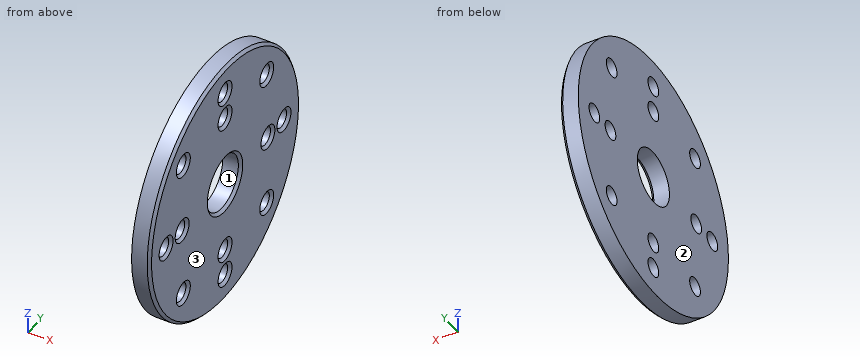
```python
from build123d import *

# Parameters (mm, degrees)
SKETCH1_W          = 2
SKETCH1_H          = 11
SKETCH2_R          = 1
CUT_EXTRUDE1_DEPTH = 20.899748742
CIRPATTERN2_COUNT  = 8
SKETCH3_R          = 1
CUT_EXTRUDE2_DEPTH = 20.899748742
CIRPATTERN3_COUNT  = 4
CHAMFER1_SIZE      = 0.3


with BuildPart() as part:
    # Sketch1 → Revolve1 (revolve)
    with BuildSketch(Plane.XY, mode=Mode.PRIVATE) as revolve1_sk:
        with Locations((-1, 8.5)):
            Rectangle(SKETCH1_W, SKETCH1_H)
    revolve(revolve1_sk.sketch.rotate(Axis((0, 0, 0), (1, 0, 0)), 90), axis=Axis((0, 0, 0), (1, 0, 0)))

    # Sketch2 → Cut-Extrude1 (cut, through all)
    with BuildSketch(Plane(origin=(0, 0, 0), x_dir=(0, 0, -1), z_dir=(1, 0, 0))):
        with Locations((0, 11)):
            Circle(SKETCH2_R)
    cut_extrude1 = extrude(amount=-CUT_EXTRUDE1_DEPTH, mode=Mode.SUBTRACT)

    # CirPattern2: Cut-Extrude1 ×8 about axis
    cirpattern2_axis = Axis((0, 0, 0), (1, 0, 0))
    for i in range(1, CIRPATTERN2_COUNT):
        add(cut_extrude1.rotate(cirpattern2_axis, i * 360 / CIRPATTERN2_COUNT), mode=Mode.SUBTRACT)

    # Sketch3 → Cut-Extrude2 (cut, through all)
    with BuildSketch(Plane(origin=(0, 0, 0), x_dir=(0, 0, -1), z_dir=(1, 0, 0))):
        with Locations((0, 8)):
            Circle(SKETCH3_R)
    cut_extrude2 = extrude(amount=-CUT_EXTRUDE2_DEPTH, mode=Mode.SUBTRACT)

    # CirPattern3: Cut-Extrude2 ×4 about axis
    cirpattern3_axis = Axis((0, 0, 0), (1, 0, 0))
    for i in range(1, CIRPATTERN3_COUNT):
        add(cut_extrude2.rotate(cirpattern3_axis, i * 360 / CIRPATTERN3_COUNT), mode=Mode.SUBTRACT)

    # Chamfer1
    chamfer1_edges = [part.edges().sort_by_distance(p)[0] for p in [
        (0, 11, 1),
        (0, 8.485281374, -7.071067812),
        (0, 1, -11),
        (0, -7.071067812, -8.485281374),
        (0, -11, -1),
        (0, -8.485281374, 7.071067812),
        (0, -1, 11),
        (0, 0, -3),
        (0, 7.071067812, 8.485281374),
        (0, 0, -14),
        (0, 8, 1),
        (0, 1, -8),
        (0, -8, -1),
        (0, -1, 8),
    ]]
    chamfer(chamfer1_edges, length=CHAMFER1_SIZE)


solid = part.part
```
Geometry check sheet. Reference: the model listing, model coordinates, mm. Face numbers are marked on the shaded views. Round coordinates to 2 decimals unless told otherwise and drop trailing zeros. Answer as CSV lines item,"result".
1) Sectioned sample at A-A on x = -0.7. Give the number of separate pieces and of enclosed holes in the cut face, and give its area (3 significant figures).
Entries:
separate pieces,"1"
enclosed holes,"13"
area,"550 mm2"
2) Gauge pin test, flat ends, axial feed: pin 1 Ø2.5 at (y, z) = (0, 8) entering from +X; pin 2 Ø1 at (x, y) = (-1, 8) entering from -Z. Record the tip position at first contact, or that the pin passes through.
Entries:
pin 1,"x = -0.05"
pin 2,"z = -11.82"
3) Mould release check, pull along X, two halves, no side actions. Record for the marked faces 1, 2 and 3: +X half, -X half, draft (parallel to the pull), parting line (faces both ways), or undercut.
Entries:
face 1,"draft"
face 2,"-X half"
face 3,"+X half"
4) Thickness scan on probe 1 along Y at (x, z) = (-1.4, 0); probe 2 along Z at (x, y) = (-1.9, 8.25); probe 3 along Z at (x, y) = (-1.6, -8). Record the ranges inside material, lowest first. Write a range as [from, to].
Entries:
probe 1,"[-14, -12], [-10, -9], [-7, -3], [3, 7], [9, 10], [12, 14]"
probe 2,"[-11.31, -8.66], [-6.9, -0.97], [0.97, 6.9], [8.66, 11.31]"
probe 3,"[-11.49, -8.75], [-6.8, -1], [1, 6.8], [8.75, 11.49]"
